CAD build for the part. Positions are in the model's coordinates, mm. Face numbers are marked on the shaded views. A direction names the side the tool comes from. Coordinates: 2 decimals unless noted, no trailing zeros. Loops run counter-clockwise (first coordinate to the right, second up) from the corner with the lowest first, then second, coordinate; pieces in that order, holes last. Notation, with made-up numbers: (54, 50.25) - (60, 50.25) arc R14 ccw to (60, 71.25) - close; hole circle Ø7 at (30.5, -15). An arc over 180 degrees is marked (long way). Put each result on its own line as item: value.
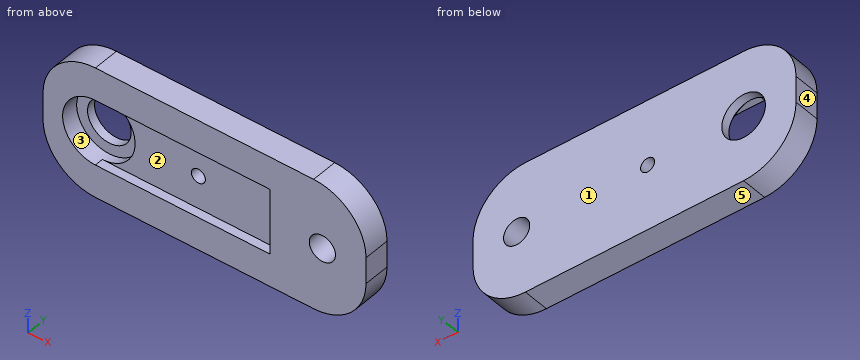
```python
from build123d import *

# Parameters (mm, degrees)
SKETCH1_W           = 30
SKETCH1_H           = 15
BOSS_EXTRUDE2_DEPTH = 3
CUT_EXTRUDE1_REACH  = 19.037
SKETCH3_R           = 2.5
FILLET1_R           = 6
SKETCH5_W           = 12
SKETCH5_H           = 3
BOSS_EXTRUDE3_DEPTH = 10
SKETCH6_R           = 3.75
CUT_EXTRUDE4_DEPTH  = 2
SKETCH7_W           = 20
SKETCH7_H           = 7.5
CUT_EXTRUDE5_DEPTH  = 1
CUT_EXTRUDE6_REACH  = 25.135
SKETCH8_R           = 0.8
CUT_EXTRUDE7_REACH  = 25.243
SKETCH9_W           = 12
SKETCH9_H           = 10
SKETCH10_W          = 15
SKETCH10_H          = 3
BOSS_EXTRUDE4_DEPTH = 7
CUT_EXTRUDE8_REACH  = 25.436
SKETCH11_R          = 1.5
FILLET2_R           = 6


with BuildPart() as part:
    # Sketch1 → Boss-Extrude2 (new body)
    with BuildSketch(Plane(origin=(0, 0, 0), x_dir=(1, 0, 0), z_dir=(0, 1, 0))):
        Rectangle(SKETCH1_W, SKETCH1_H)
    extrude(amount=BOSS_EXTRUDE2_DEPTH)

    # Sketch3 → Cut-Extrude1 (cut, up to next)
    with BuildSketch(Plane(origin=(0, 3, 0), x_dir=(1, 0, 0), z_dir=(0, 1, 0)), mode=Mode.PRIVATE) as cut_extrude1_sk1:
        with Locations(Location((-9, 0, 0), (0, 0, 270))):
            Circle(SKETCH3_R)
    cut_extrude1_tool1 = extrude(cut_extrude1_sk1.sketch, amount=-CUT_EXTRUDE1_REACH, mode=Mode.PRIVATE) & part.part
    add(cut_extrude1_tool1.solids().sort_by_distance((-9, 3, 0))[0], mode=Mode.SUBTRACT)

    # Fillet1
    fillet1_edges = [part.edges().sort_by_distance(p)[0] for p in [
        (-15, 1.5, 7.5),
        (-15, 1.5, -7.5),
    ]]
    fillet(fillet1_edges, radius=FILLET1_R)

    # Sketch5 → Boss-Extrude3 (add)
    with BuildSketch(Plane.XY.offset(7.5)):
        with Locations((9, 1.5)):
            Rectangle(SKETCH5_W, SKETCH5_H)
    extrude(amount=BOSS_EXTRUDE3_DEPTH)

    # Sketch6 → Cut-Extrude4 (cut)
    with BuildSketch(Plane(origin=(0, 0, 0), x_dir=(-1, 0, 0), z_dir=(0, -1, 0))):
        with Locations(Location((9, 0, 0), (0, 0, 90))):
            Circle(SKETCH6_R)
    extrude(amount=-CUT_EXTRUDE4_DEPTH, mode=Mode.SUBTRACT)

    # Sketch7 → Cut-Extrude5 (cut)
    with BuildSketch(Plane(origin=(0, 0, 0), x_dir=(-1, 0, 0), z_dir=(0, -1, 0))):
        with Locations((-1, 0)):
            Rectangle(SKETCH7_W, SKETCH7_H)
    extrude(amount=-CUT_EXTRUDE5_DEPTH, mode=Mode.SUBTRACT)

    # Sketch8 → Cut-Extrude6 (cut, up to next)
    with BuildSketch(Plane(origin=(0, 1, 0), x_dir=(-1, 0, 0), z_dir=(0, -1, 0)), mode=Mode.PRIVATE) as cut_extrude6_sk1:
        with Locations(Location((-2, 0, 0), (0, 0, 90))):
            Circle(SKETCH8_R)
    cut_extrude6_tool1 = extrude(cut_extrude6_sk1.sketch, amount=-CUT_EXTRUDE6_REACH, mode=Mode.PRIVATE) & part.part
    add(cut_extrude6_tool1.solids().sort_by_distance((2, 1, 0))[0], mode=Mode.SUBTRACT)

    # Sketch9 → Cut-Extrude7 (cut, up to next)
    with BuildSketch(Plane(origin=(0, 0, 0), x_dir=(1, 0, 0), z_dir=(0, 1, 0)), mode=Mode.PRIVATE) as cut_extrude7_sk1:
        with Locations((9, -12.5)):
            Rectangle(SKETCH9_W, SKETCH9_H)
    cut_extrude7_tool1 = extrude(cut_extrude7_sk1.sketch, amount=CUT_EXTRUDE7_REACH, mode=Mode.PRIVATE) & part.part
    add(cut_extrude7_tool1.solids().sort_by_distance((9, 0, 12.5))[0], mode=Mode.SUBTRACT)

    # Sketch10 → Boss-Extrude4 (add)
    with BuildSketch(Plane(origin=(15, 0, 0), x_dir=(0, 0, -1), z_dir=(1, 0, 0))):
        with Locations((0, 1.5)):
            Rectangle(SKETCH10_W, SKETCH10_H)
    extrude(amount=BOSS_EXTRUDE4_DEPTH)

    # Sketch11 → Cut-Extrude8 (cut, up to next)
    with BuildSketch(Plane(origin=(0, 3, 0), x_dir=(1, 0, 0), z_dir=(0, 1, 0)), mode=Mode.PRIVATE) as cut_extrude8_sk1:
        with Locations(Location((17, 0, 0), (0, 0, 270))):
            Circle(SKETCH11_R)
    cut_extrude8_tool1 = extrude(cut_extrude8_sk1.sketch, amount=-CUT_EXTRUDE8_REACH, mode=Mode.PRIVATE) & part.part
    add(cut_extrude8_tool1.solids().sort_by_distance((17, 3, 0))[0], mode=Mode.SUBTRACT)

    # Fillet2
    fillet2_edges = [part.edges().sort_by_distance(p)[0] for p in [
        (22, 1.5, -7.5),
        (22, 1.5, 7.5),
    ]]
    fillet(fillet2_edges, radius=FILLET2_R)


solid = part.part
```
Q1. Slice it at B-B, the plane x = 2. Give the cut face in (y, z), then the cut area to 3 significant figures.
Determined:
outline: (0, -7.5) - (3, -7.5) - (3, -0.8) - (1, -0.8) - (1, -3.75) - (0, -3.75) - close; (0, 3.75) - (1, 3.75) - (1, 0.8) - (3, 0.8) - (3, 7.5) - (0, 7.5) - close
area: 34.3 mm2
Q2. Slice it at D-D, the plane x = -2. Give the cut face in (y, z).
Determined:
outline: (0, -7.5) - (3, -7.5) - (3, 7.5) - (0, 7.5) - (0, 3.75) - (1, 3.75) - (1, -3.75) - (0, -3.75) - close
Q3. Wall check: L1, parallel to X at y = 1.1, z = 0; L2, parallel to X at y = 2.4, z = 0; L3, parallel to Z at x = -9, y = 1. Give the ranges that are in metal, low to high. Write a range as from..to.
Determined:
L1: -15..-12.75, -5.25..1.2, 2.8..15.5, 18.5..22
L2: -15..-11.5, -6.5..1.2, 2.8..15.5, 18.5..22
L3: -7.5..-3.75, 3.75..7.5
Q4. Slice it at A-A, the plane z = 0. Give the cut face in (x, y).
Determined:
outline: (-15, 0) - (-12.75, 0) - (-12.75, 2) - (-11.5, 2) - (-11.5, 3) - (-15, 3) - close; (-6.5, 2) - (-5.25, 2) - (-5.25, 1) - (1.2, 1) - (1.2, 3) - (-6.5, 3) - close; (2.8, 1) - (11, 1) - (11, 0) - (15.5, 0) - (15.5, 3) - (2.8, 3) - close; (18.5, 0) - (22, 0) - (22, 3) - (18.5, 3) - close
Q5. Tool access for the marked faces 1 and 2: list every direction of +Z, -Z, +X, -X, +Y, -Y with a clear straight run to the whole face (end or side of a thin tool).
Determined:
face 1: +Z, -Z, +X, -X, +Y
face 2: -Y
Q6. Pin check, flat tips, straight feed: pin 1 Ø4 at (x, z) = (-9, 0) entering from +Y; pin 2 Ø8 at (x, z) = (-9.5, 0.5) entering from -Y; pin 3 Ø2 at (x, z) = (0.5, 2) entering from -Y. Stop position of each tip, or through.
Determined:
pin 1: through
pin 2: y = 0
pin 3: y = 1
Q7. Mould opens along Z. For the marked faces 3, 4 and 5 say: +Z half, -Z half, draft (parallel to the pull), parting line (faces both ways), or undercut.
Determined:
face 3: undercut
face 4: draft
face 5: -Z half
Q8. Slice it at C-C, the plane z = 2. Give the cut face in (x, y).
Determined:
outline: (-14.98, 0) - (-12.17, 0) - (-12.17, 2) - (-10.5, 2) - (-10.5, 3) - (-14.98, 3) - close; (-7.5, 2) - (-5.83, 2) - (-5.83, 1) - (11, 1) - (11, 0) - (21.98, 0) - (21.98, 3) - (-7.5, 3) - close
